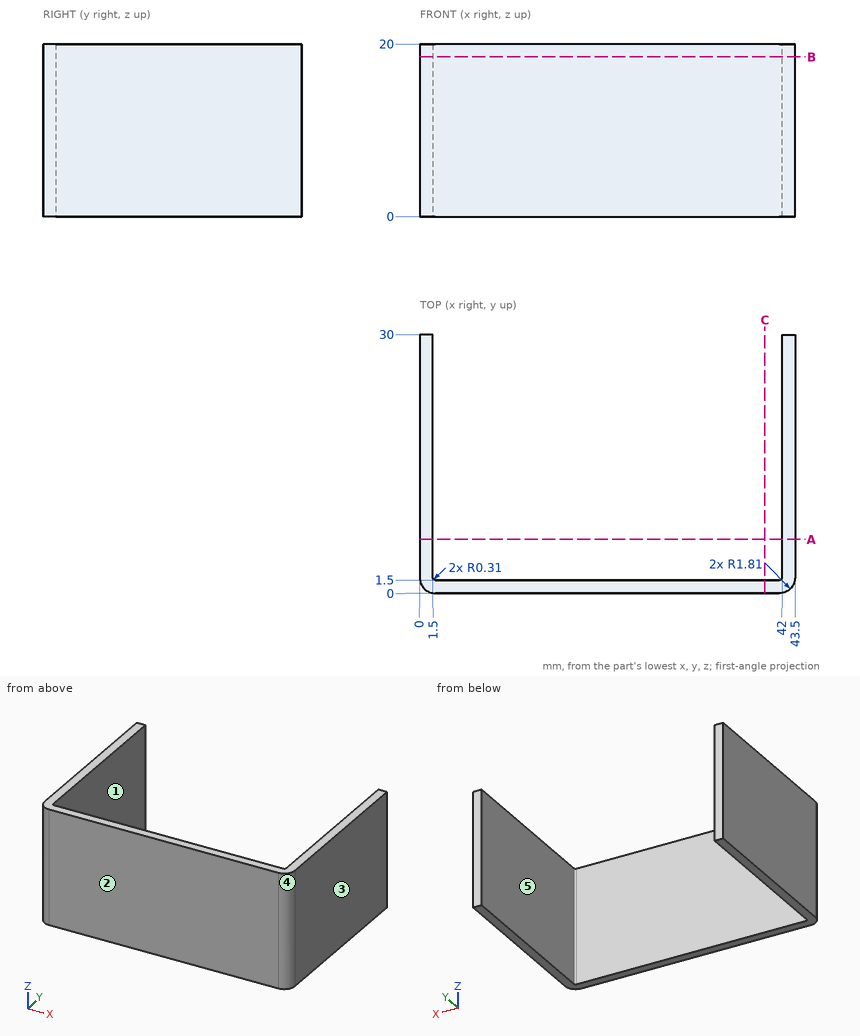
Source: three-view drawing plus pictorial views. Frame: mm from the lowest corner of the part. A direction names the side the tool comes from. Coordinates: 2 decimals unless noted, no trailing zeros. Loops run counter-clockwise (first coordinate to the right, second up) from the corner with the lowest first, then second, coordinate; pieces in that order, holes last. Notation, with made-up numbers: (3.5, -37.5) -> (12.5, -37.5) arc R15 ccw to (12.5, -13.5) -> close; hole circle Ø4 at (-31.75, 2). An arc over 180 degrees is marked (long way). Write each question's results on one line, items separated by ' | '. Start each with the question number.
Q1. Pin query (flat end, axial travel): pin 1 (1.5 mm diameter, centred on x = 31.5, z = 14, fed in from +Y); pin 2 (5 mm diameter, centred on x = 39, y = 11.5, fed in from +Z). Return the tip coordinate at first contact, or that it passes through.
Q2. Section A-A, the plane y = 6.25. Return the cut outline in (x, z).
Q3. Section B-B, the plane z = 18.5. Return the cut outline in (x, y), plus the area to 3 significant figures.
Q4. Pull-direction query (X, two-part tool) for the marked faces 1, 2 and 3; classes: released by +X, released by -X, zero draft, split by the parting line, or undercut.
Q5. Ray query, line 1 (X direction, y = 1.75, z = 16); line 2 (Y direction, x = 37, z = 3.75). Return the intervals inside material, ascending. Write a range as from..to.
Q6. Reachability of the marked faces 4 and 5 from +Z, -Z, +X, -X, +Y, -Y: full face, straight path, thin tool, end or side. Return the list, or none.
Q7. Section C-C, the plane x = 40. Return the cut outline in (y, z).
Found:
1) pin 1: y = 1.5 | pin 2: through
2) outline: (0, 0) -> (1.5, 0) -> (1.5, 20) -> (0, 20) -> close; (42, 0) -> (43.5, 0) -> (43.5, 20) -> (42, 20) -> close
3) outline: (0, 1.81) arc R1.81 ccw to (1.81, 0) -> (41.69, 0) arc R1.81 ccw to (43.5, 1.81) -> (43.5, 30) -> (42, 30) -> (42, 1.81) arc R0.31 cw to (41.69, 1.5) -> (1.81, 1.5) arc R0.31 cw to (1.5, 1.81) -> (1.5, 30) -> (0, 30) -> close | area: 149 mm2
4) face 1: undercut | face 2: zero draft | face 3: released by +X
5) line 1: 0..1.51, 41.99..43.5 | line 2: 0..1.5
6) face 4: +Z, -Z, +X, -Y | face 5: +Z, -Z, +Y
7) outline: (0, 0) -> (1.5, 0) -> (1.5, 20) -> (0, 20) -> close
